Answer from the drawing. Dimensions are ordinates in mm from the lowest x, y and z of the part. Give positions to 0.01 mm unless a question says otherwise; leave off trailing zeros. Loops run counter-clockwise (first coordinate to the right, second up) from the corner with the lowest first, then second, coordinate; pieces in that order, holes last. Notation, with made-up numbers: M -22,57.5 L -14,57.5 A18 cw -14,61.5 Z; hole C -23.5,21 d6. An arc over 180 degrees is marked long. Use a Markdown table: item, result.
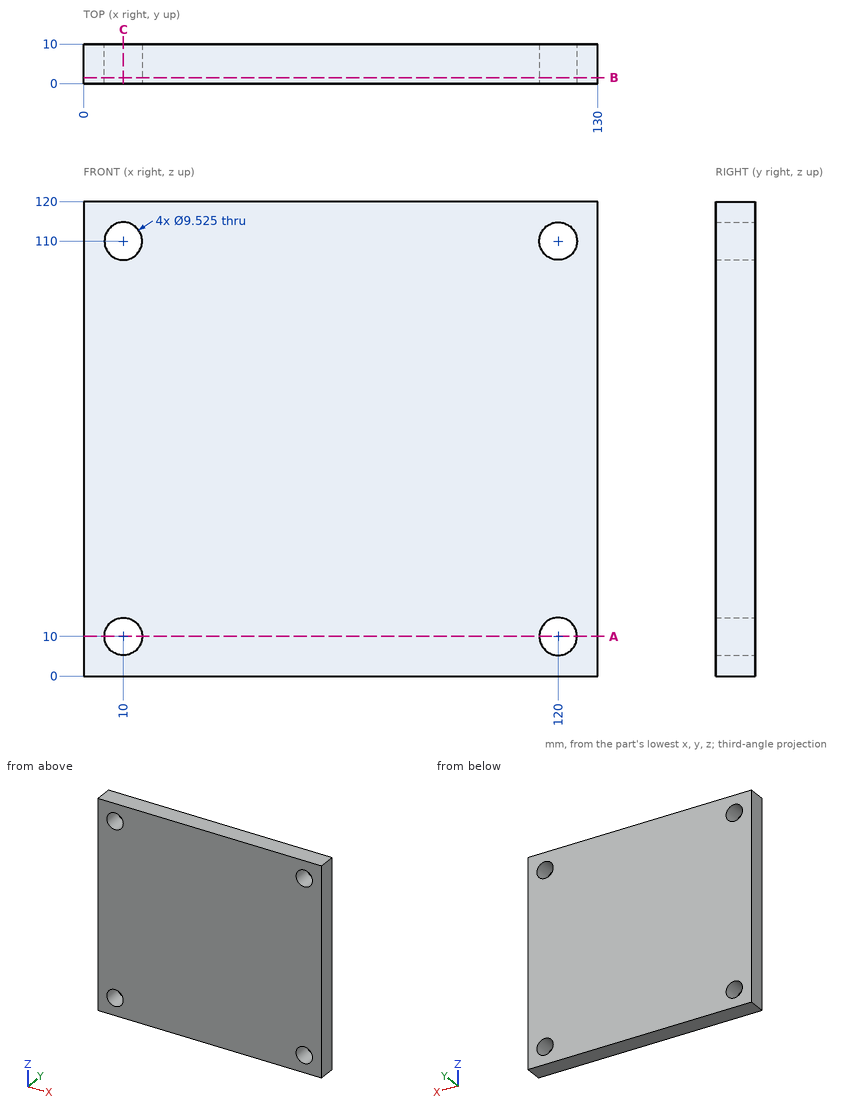
(1) A cutting plane is placed at C-C (x = 10). Write down the section's boundary in (y, z), and give its area (3 significant figures).
Entries:
| item | result |
|---|---|
| outline | M 0,0 L 10,0 L 10,5.24 L 0,5.24 Z; M 0,14.76 L 10,14.76 L 10,105.24 L 0,105.24 Z; M 0,114.76 L 10,114.76 L 10,120 L 0,120 Z |
| area | 1,010 mm² |
(2) A cutting plane is placed at B-B (y = 1.5). Write down the section's boundary in (x, z) (1 decimal), and give its area (3 significant figures).
Entries:
| item | result |
|---|---|
| outline | M 0,0 L 130,0 L 130,120 L 0,120 Z; hole C 10,10 d9.5; hole C 10,110 d9.5; hole C 120,10 d9.5; hole C 120,110 d9.5 |
| area | 15,300 mm² |
(3) Given P1, Ø2, axis at x = 26, z = 66.5, coming from the -Y side; P2, Ø8.5, axis at x = 120, z = 110, coming from the +Y side, each flat-ended and moving along its own axis, determine where each tip first touches the part or whether it passes through.
Entries:
| item | result |
|---|---|
| P1 | stops at y = 0 |
| P2 | passes through |
(4) A cutting plane is placed at A-A (z = 10). Write down the section's boundary in (x, y), and give its area (3 significant figures).
Entries:
| item | result |
|---|---|
| outline | M 0,0 L 5.24,0 L 5.24,10 L 0,10 Z; M 14.76,0 L 115.24,0 L 115.24,10 L 14.76,10 Z; M 124.76,0 L 130,0 L 130,10 L 124.76,10 Z |
| area | 1,110 mm² |
(5) Consider probe 1 along Z at (x, y) = (10, 3.5); probe 2 along X at (y, z) = (4, 10); probe 3 along X at (y, z) = (8.5, 107). Determine where each line is inside the solid, lowest interval first. Write a range as [from, to].
Entries:
| item | result |
|---|---|
| probe 1 | z = [0, 5.24], [14.76, 105.24], [114.76, 120] |
| probe 2 | x = [0, 5.24], [14.76, 115.24], [124.76, 130] |
| probe 3 | x = [0, 6.3], [13.7, 116.3], [123.7, 130] |
